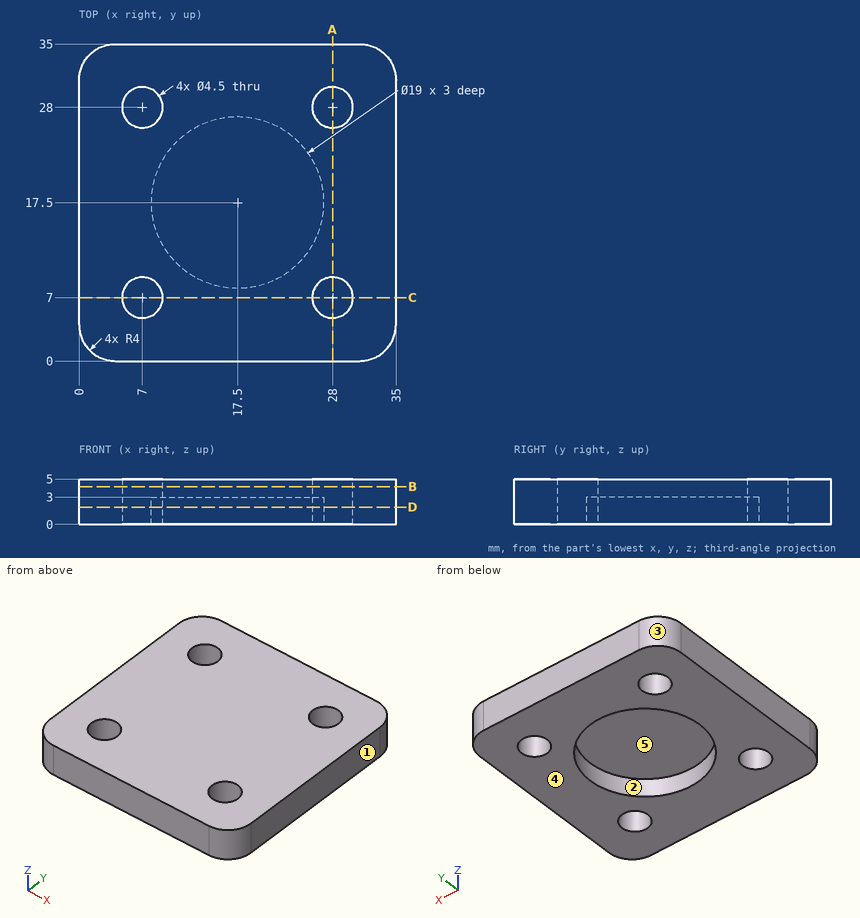
Geometry check sheet. Reference: drawing and pictorial views, mm from the part's lowest x, y, z. A direction names the side the tool comes from. Give positions to 0.01 mm unless a question says otherwise; leave off trailing zeros. Order: outer loops, then holes, each group sorted by start corner. A loop starts at its lowest first (then second) coordinate and runs counter-clockwise, first axis right, second up. Notation, with made-up numbers: M -36.5,0 L -18.5,0 A22 cw -18.5,13 Z; hole C 23.25,33 d8. An arc over 180 degrees is marked long. Return JSON: item names as keys, results as strings. Group by question number.
1) Section check B-B on z = 4.15. Record the cut outline in (x, y).
2) Access from +Z, -Z, +X, -X, +Y, -Y to the whole of each face (thin tool, end or side, straight path). Record for the marked faces 4 and 5.
3) Section check A-A on x = 28. Record the cut outline in (y, z), and give its area (3 significant figures).
4) Section check D-D on z = 1.9. Record the cut outline in (x, y), and give its area (3 significant figures).
5) Go/stop test with flat-tipped pins: pin 1 Ø2.5 at (x, y) = (28, 7) entering from +Z; pin 2 Ø11.5 at (x, y) = (17.5, 17.5) entering from -Z. Record where each tip stops, or that it passes through.
6) Scan lines: line 1 (Y direction, x = 7, z = 2); line 2 (X direction, y = 5.5, z = 3.2). Record each from-to range of solid material in increasing order.
7) Mould release check, pull along X, two halves, no side actions. Record for the marked faces 1, 2 and 3: pulls with the +X half, pulls with the -X half, needs draft (parallel to the pull), parting line crosses it, or undercut.
Answer block:
{
 "1": {"outline": "M 0,4 A4 ccw 4,0 L 31,0 A4 ccw 35,4 L 35,31 A4 ccw 31,35 L 4,35 A4 ccw 0,31 Z; hole C 7,7 d4.5; hole C 7,28 d4.5; hole C 28,7 d4.5; hole C 28,28 d4.5"},
 "2": {"face 4": "-Z, +X, -X, +Y, -Y", "face 5": "-Z"},
 "3": {"outline": "M 0,0 L 4.75,0 L 4.75,5 L 0,5 Z; M 9.25,0 L 25.75,0 L 25.75,5 L 9.25,5 Z; M 30.25,0 L 35,0 L 35,5 L 30.25,5 Z", "area": "130 mm^2"},
 "4": {"outline": "M 0,4 A4 ccw 4,0 L 31,0 A4 ccw 35,4 L 35,31 A4 ccw 31,35 L 4,35 A4 ccw 0,31 Z; hole C 7,7 d4.5; hole C 7,28 d4.5; hole C 17.5,17.5 d19; hole C 28,7 d4.5; hole C 28,28 d4.5", "area": "864 mm^2"},
 "5": {"pin 1": "passes through", "pin 2": "stops at z = 3"},
 "6": {"line 1": "y = 0 to 4.75, 9.25 to 25.75, 30.25 to 35", "line 2": "x = 0 to 5.32, 8.68 to 26.32, 29.68 to 35"},
 "7": {"face 1": "pulls with the +X half", "face 2": "undercut", "face 3": "pulls with the -X half"}
}
